Work out the finished part from the listing and answer in its coordinate system (mm). Face numbers are marked on the shaded views. A direction names the side the tool comes from. Round coordinates to 2 decimals unless told otherwise and drop trailing zeros. Loops run counter-clockwise (first coordinate to the right, second up) from the corner with the lowest first, then second, coordinate; pieces in that order, holes last. Notation, with made-up numbers: (-7.75, 58.25) -> (40.25, 58.25) arc R8 ccw to (40.25, 67.25) -> close; hole circle Ø6 at (43, -8). An arc over 180 degrees is marked (long way). Use one line per item in the form item = value.
```python
from build123d import *

# Parameters (mm, degrees)
SKETCH_1_R                       = 150
EXTRUDE_1_DEPTH                  = 34.5
EXTRUDE_2_DEPTH                  = 130
SKETCH_3_R                       = 48.25
CUT_EXTRUDE_1_DEPTH              = 314.765836254
SKETCH_4_R                       = 90
CUT_EXTRUDE_2_DEPTH              = 24.5
SKETCH_6_R                       = 48.25
EXTRUDE_3_DEPTH                  = 5
PATTERN_LINEAR_1_COUNT           = 2
PATTERN_LINEAR_1_PITCH           = 221
SKETCH_10_R                      = 32
CUT_EXTRUDE_3_DEPTH              = 5
SKETCH_11_R                      = 1
CUT_EXTRUDE_4_DEPTH              = 5
PATTERN_CIRCULAR_1_COUNT         = 8
PATTERN_LINEAR_3_COUNT           = 2
PATTERN_LINEAR_3_PITCH           = 221
PATTERN_LINEAR_3_COPY_1_SKETCH_R = 1
PATTERN_LINEAR_3_COPY_1_DEPTH    = 5
PATTERN_LINEAR_3_COPY_2_SKETCH_R = 1
PATTERN_LINEAR_3_COPY_2_DEPTH    = 5
PATTERN_LINEAR_3_COPY_3_SKETCH_R = 1
PATTERN_LINEAR_3_COPY_3_DEPTH    = 5
PATTERN_LINEAR_3_COPY_4_SKETCH_R = 1
PATTERN_LINEAR_3_COPY_4_DEPTH    = 5
PATTERN_LINEAR_3_COPY_5_SKETCH_R = 1
PATTERN_LINEAR_3_COPY_5_DEPTH    = 5
PATTERN_LINEAR_3_COPY_6_SKETCH_R = 1
PATTERN_LINEAR_3_COPY_6_DEPTH    = 5
PATTERN_LINEAR_3_COPY_7_SKETCH_R = 1
PATTERN_LINEAR_3_COPY_7_DEPTH    = 5
PATTERN_LINEAR_4_COUNT           = 2
PATTERN_LINEAR_4_PITCH           = 221
SKETCH_14_R                      = 3
CUT_EXTRUDE_5_DEPTH              = 249.797106092
SKETCH_16_R                      = 2
CUT_EXTRUDE_6_DEPTH              = 255.165300543
PATTERN_CIRCULAR_2_COUNT         = 6
SKETCH_17_R                      = 36
CUT_EXTRUDE_7_DEPTH              = 10


with BuildPart() as part:
    # 草图1 → 凸台-拉伸1 (new body)
    with BuildSketch(Plane(origin=(0, 0, 0), x_dir=(1, 0, 0), z_dir=(0, 1, 0))):
        with Locations(Location((0, 0, 0), (0, 0, 270))):
            Circle(SKETCH_1_R)
    extrude(amount=EXTRUDE_1_DEPTH)

    # 草图2 → 凸台-拉伸2 (add)
    with BuildSketch(Plane(origin=(0, 0, 0), x_dir=(-1, 0, 0), z_dir=(0, -1, 0))):
        Polygon((100, 0), (100, 60), (133, 60), (133, -60), (100, -60), align=None)
        Polygon((-60, 0), (-60, 60), (-93, 60), (-93, -60), (-60, -60), align=None)
    extrude(amount=EXTRUDE_2_DEPTH)

    # 草图3 → 切除-拉伸1 (cut, through all)
    with BuildSketch(Plane(origin=(93, 0, 0), x_dir=(0, 0, -1), z_dir=(1, 0, 0))):
        with Locations((0, -70)):
            Circle(SKETCH_3_R)
    extrude(amount=-CUT_EXTRUDE_1_DEPTH, mode=Mode.SUBTRACT)

    # 草图4 → 切除-拉伸2 (cut)
    with BuildSketch(Plane(origin=(0, 34.5, 0), x_dir=(1, 0, 0), z_dir=(0, 1, 0))):
        with Locations(Location((0, 0, 0), (0, 0, 270))):
            Circle(SKETCH_4_R)
    extrude(amount=-CUT_EXTRUDE_2_DEPTH, mode=Mode.SUBTRACT)

    # 草图6 → 凸台-拉伸3 (add)
    with BuildSketch(Plane(origin=(93, 0, 0), x_dir=(0, 0, -1), z_dir=(1, 0, 0))):
        with Locations((0, -70)):
            Circle(SKETCH_6_R)
    extrude_3 = extrude(amount=-EXTRUDE_3_DEPTH)

    # 阵列(线性)1: 凸台-拉伸3 ×2
    with Locations(*[(-i * PATTERN_LINEAR_1_PITCH, 0, 0) for i in range(1, PATTERN_LINEAR_1_COUNT)]):
        add(extrude_3)

    # 草图10 → 切除-拉伸3 (cut)
    with BuildSketch(Plane(origin=(93, 0, 0), x_dir=(0, 0, -1), z_dir=(1, 0, 0))):
        with Locations((0, -70)):
            Circle(SKETCH_10_R)
    cut_extrude_3 = extrude(amount=-CUT_EXTRUDE_3_DEPTH, mode=Mode.SUBTRACT)

    # 草图11 → 切除-拉伸4 (cut)
    with BuildSketch(Plane(origin=(93, 0, 0), x_dir=(0, 0, -1), z_dir=(1, 0, 0))):
        with Locations((0, -27.5)):
            Circle(SKETCH_11_R)
    cut_extrude_4 = extrude(amount=-CUT_EXTRUDE_4_DEPTH, mode=Mode.SUBTRACT)

    # 阵列(圆周)1: 切除-拉伸4 ×8 about axis
    pattern_circular_1_axis = Axis((0, -70, 0), (1, 0, 0))
    for i in range(1, PATTERN_CIRCULAR_1_COUNT):
        add(cut_extrude_4.rotate(pattern_circular_1_axis, i * 360 / PATTERN_CIRCULAR_1_COUNT), mode=Mode.SUBTRACT)

    # 阵列(线性)3: 切除-拉伸4 ×2
    with Locations(*[(-i * PATTERN_LINEAR_3_PITCH, 0, 0) for i in range(1, PATTERN_LINEAR_3_COUNT)]):
        add(cut_extrude_4, mode=Mode.SUBTRACT)

    # 阵列(线性)3 copy 1 sketch → 阵列(线性)3 copy 1 (cut)
    with BuildSketch(Plane(origin=(-128, -20.502525317, 49.497474683), x_dir=(0, 0.7071067811865475, -0.7071067811865476), z_dir=(1, 0, 0))):
        with Locations((0, -27.5)):
            Circle(PATTERN_LINEAR_3_COPY_1_SKETCH_R)
    extrude(amount=-PATTERN_LINEAR_3_COPY_1_DEPTH, mode=Mode.SUBTRACT)

    # 阵列(线性)3 copy 2 sketch → 阵列(线性)3 copy 2 (cut)
    with BuildSketch(Plane(origin=(-128, -70, 70), x_dir=(0, 1, 0), z_dir=(1, 0, 0))):
        with Locations((0, -27.5)):
            Circle(PATTERN_LINEAR_3_COPY_2_SKETCH_R)
    extrude(amount=-PATTERN_LINEAR_3_COPY_2_DEPTH, mode=Mode.SUBTRACT)

    # 阵列(线性)3 copy 3 sketch → 阵列(线性)3 copy 3 (cut)
    with BuildSketch(Plane(origin=(-128, -119.497474683, 49.497474683), x_dir=(0, 0.7071067811865476, 0.7071067811865475), z_dir=(1, 0, 0))):
        with Locations((0, -27.5)):
            Circle(PATTERN_LINEAR_3_COPY_3_SKETCH_R)
    extrude(amount=-PATTERN_LINEAR_3_COPY_3_DEPTH, mode=Mode.SUBTRACT)

    # 阵列(线性)3 copy 4 sketch → 阵列(线性)3 copy 4 (cut)
    with BuildSketch(Plane(origin=(-128, -140, 0), x_dir=(0, 0, 1), z_dir=(1, 0, 0))):
        with Locations((0, -27.5)):
            Circle(PATTERN_LINEAR_3_COPY_4_SKETCH_R)
    extrude(amount=-PATTERN_LINEAR_3_COPY_4_DEPTH, mode=Mode.SUBTRACT)

    # 阵列(线性)3 copy 5 sketch → 阵列(线性)3 copy 5 (cut)
    with BuildSketch(Plane(origin=(-128, -119.497474683, -49.497474683), x_dir=(0, -0.7071067811865475, 0.7071067811865477), z_dir=(1, 0, 0))):
        with Locations((0, -27.5)):
            Circle(PATTERN_LINEAR_3_COPY_5_SKETCH_R)
    extrude(amount=-PATTERN_LINEAR_3_COPY_5_DEPTH, mode=Mode.SUBTRACT)

    # 阵列(线性)3 copy 6 sketch → 阵列(线性)3 copy 6 (cut)
    with BuildSketch(Plane(origin=(-128, -70, -70), x_dir=(0, -1, 0), z_dir=(1, 0, 0))):
        with Locations((0, -27.5)):
            Circle(PATTERN_LINEAR_3_COPY_6_SKETCH_R)
    extrude(amount=-PATTERN_LINEAR_3_COPY_6_DEPTH, mode=Mode.SUBTRACT)

    # 阵列(线性)3 copy 7 sketch → 阵列(线性)3 copy 7 (cut)
    with BuildSketch(Plane(origin=(-128, -20.502525317, -49.497474683), x_dir=(0, -0.7071067811865477, -0.7071067811865474), z_dir=(1, 0, 0))):
        with Locations((0, -27.5)):
            Circle(PATTERN_LINEAR_3_COPY_7_SKETCH_R)
    extrude(amount=-PATTERN_LINEAR_3_COPY_7_DEPTH, mode=Mode.SUBTRACT)

    # 阵列(线性)4: 切除-拉伸3 ×2
    with Locations(*[(-i * PATTERN_LINEAR_4_PITCH, 0, 0) for i in range(1, PATTERN_LINEAR_4_COUNT)]):
        add(cut_extrude_3, mode=Mode.SUBTRACT)

    # 草图14 → 切除-拉伸5 (cut, through all)
    with BuildSketch(Plane.XZ):
        with Locations(Location((-77.76, -100, 0), (0, 0, 270))):
            Circle(SKETCH_14_R)
    cut_extrude_5 = extrude(amount=-CUT_EXTRUDE_5_DEPTH, mode=Mode.SUBTRACT)

    # 镜向1: 切除-拉伸5 across plane
    add(cut_extrude_5.mirror(Plane.XY), mode=Mode.SUBTRACT)

    # 草图16 → 切除-拉伸6 (cut, through all)
    with BuildSketch(Plane(origin=(0, 10, 0), x_dir=(1, 0, 0), z_dir=(0, 1, 0))):
        with Locations(Location((0, 34.5, 0), (0, 0, 270))):
            Circle(SKETCH_16_R)
    cut_extrude_6 = extrude(amount=-CUT_EXTRUDE_6_DEPTH, mode=Mode.SUBTRACT)

    # 阵列(圆周)2: 切除-拉伸6 ×6 about axis
    pattern_circular_2_axis = Axis((0, 0, 0), (0, 1, 0))
    for i in range(1, PATTERN_CIRCULAR_2_COUNT):
        add(cut_extrude_6.rotate(pattern_circular_2_axis, i * 360 / PATTERN_CIRCULAR_2_COUNT), mode=Mode.SUBTRACT)

    # 草图17 → 切除-拉伸7 (cut)
    with BuildSketch(Plane(origin=(93, 0, 0), x_dir=(0, 0, -1), z_dir=(1, 0, 0))):
        with Locations((0, -70)):
            Circle(SKETCH_17_R)
    extrude(amount=-CUT_EXTRUDE_7_DEPTH, mode=Mode.SUBTRACT)


solid = part.part
```
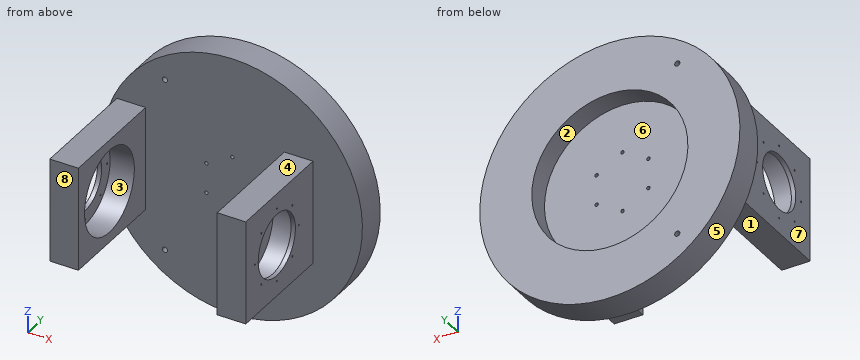
(1) Find section A-A, the plane y = -14. Write down the section's boundary in (x, z).
Completed:
outline = (-133, -60) -> (-100, -60) -> (-100, 60) -> (-133, 60) -> close; (60, -60) -> (93, -60) -> (93, 60) -> (60, 60) -> close
(2) Find section D-D, the plane y = -84. Write down the section's boundary in (x, z).
Completed:
outline = (-133, -60) -> (-100, -60) -> (-100, -46.17) -> (-128, -46.17) -> (-128, -28.77) -> (-133, -28.77) -> close; (-133, 28.77) -> (-128, 28.77) -> (-128, 46.17) -> (-100, 46.17) -> (-100, 60) -> (-133, 60) -> close; (60, -60) -> (93, -60) -> (93, -33.17) -> (88, -33.17) -> (88, -46.17) -> (60, -46.17) -> close; (60, 46.17) -> (88, 46.17) -> (88, 33.17) -> (93, 33.17) -> (93, 60) -> (60, 60) -> close
(3) Given P1, Ø2.5, axis at y = -39.95, z = 30.05, coming from the +X side; P2, Ø2.5, axis at y = -100.05, z = -30.05, coming from the -X side; P3, Ø6, axis at x = -86, z = 49, coming from the -Y side, each flat-ended and moving along its own axis, determine where each tip first touches the part or whether it passes through.
Completed:
P1 = 93
P2 = -133
P3 = 0
(4) Find section C-C, the plane z = 71. Write down the section's boundary in (x, y).
Completed:
outline = (-132.13, 0) -> (132.13, 0) -> (132.13, 34.5) -> (55.31, 34.5) -> (55.31, 10) -> (-55.31, 10) -> (-55.31, 34.5) -> (-132.13, 34.5) -> close
(5) For a pull along X with two mould halves and no side action, classify the marked faces 5, 6, 7 and 8 as +X half, -X half, draft (parallel to the pull), parting line (faces both ways), or undercut.
Completed:
face_5 = parting line
face_6 = undercut
face_7 = -X half
face_8 = draft
(6) Find section B-B, the plane x = -24. Write down the section's boundary in (y, z).
Completed:
outline = (0, -148.07) -> (34.5, -148.07) -> (34.5, -86.74) -> (10, -86.74) -> (10, 86.74) -> (34.5, 86.74) -> (34.5, 148.07) -> (0, 148.07) -> close
(7) For the marked faces 1, 2, 3 and 4, determine the directions among +Z, -Z, +X, -X, +Y, -Y from which every point of the face is accessible in a straight line to the end or side of a thin tool.
Completed:
face_1 = -Z, +X, -X, -Y
face_2 = +Y
face_3 = none
face_4 = +Z, +X, -X, -Y
(8) Consider L1, parallel to Y at x = 89.1, z = 0; L2, parallel to Y at x = 82, z = 0; L3, parallel to X at y = -21, z = 44.5. Determine where each line is inside the solid, lowest interval first.
Completed:
L1 = -130 to -113.5, -111.5 to -106, -34 to -28.5, -26.5 to 10
L2 = -130 to -118.25, -21.75 to 10
L3 = -133 to -100, 60 to 93
